Part model, mm, in its own coordinate system. Face numbers are marked on the shaded views. A direction names the side the tool comes from. Give positions to 0.01 mm unless a question says otherwise; leave off trailing zeros. Order: outer loops, then holes, each group sorted by start corner. A loop starts at its lowest first (then second) coordinate and runs counter-clockwise, first axis right, second up. Notation, with made-up numbers: (-38.75, 24.5) - (10.25, 24.5) arc R27 cw to (10.25, 48.5) - close; hole circle Ø5 at (16, 12). An arc over 180 degrees is marked (long way). Use one line per item in the form item = value. Start each with the question number.
1. Drill centre lines: line 1 (Y direction, x = -1, z = 15); line 2 (X direction, y = 2.75, z = -0.5); line 3 (X direction, y = 0.75, z = 12). Where is each one in solid material? Low to high.
2. Band-saw the part on C-C, the plane z = 15. List the corners of the cut face in (x, y), plus the area to 3 significant figures.
3. Pull direction Z, two halves, no side cores. Call the marked faces 1, 2 and 3: +Z half, -Z half, draft (parallel to the pull), parting line (faces both ways), or undercut.
4. Pin check, flat tips, straight feed: P1, Ø3, axis at y = 8.5, z = 13, coming from the +X side; P2, Ø5.5, axis at y = 5, z = 15, coming from the -X side; P3, Ø5, axis at x = 8, y = 1, coming from the +Z side; P4, Ø3, axis at x = 19.5, y = 6, coming from the -Z side. Stop position of each tip, or through.
5. Tool access for the marked faces 4, 5 and 6: list every direction of +Z, -Z, +X, -X, +Y, -Y with a clear straight run to the whole face (end or side of a thin tool).
6. Band-saw the part on B-B, the plane x = -2. List the corners of the cut face in (y, z).
7. Band-saw the part on D-D, the plane x = 15. List the corners of the cut face in (y, z), plus the area to 3 significant figures.
8. Band-saw the part on A-A, the plane y = 5. List the corners of the cut face in (x, z), plus the area to 3 significant figures.
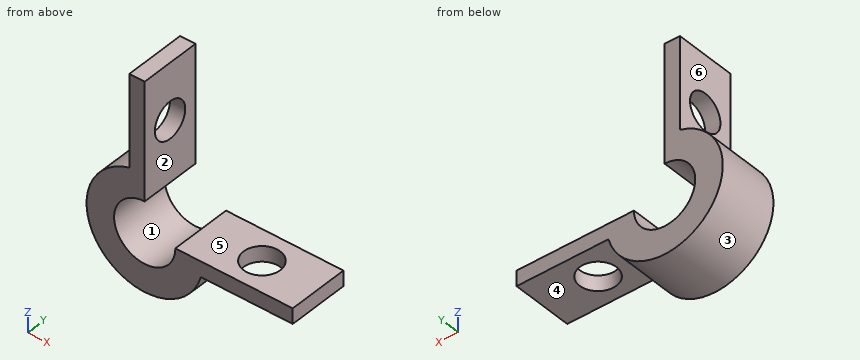
from build123d import *

# Parameters (mm, degrees)
BOSS_EXTRUDE1_DEPTH = 10
SKETCH2_R           = 3
CUT_EXTRUDE1_DEPTH  = 38.349495851
CIRPATTERN1_COUNT   = 2
CIRPATTERN1_ANGLE   = 90


with BuildPart() as part:
    # Sketch1 → Boss-Extrude1 (new body)
    with BuildSketch(Plane(origin=(0, 0, 0), x_dir=(1, 0, 0), z_dir=(0, 1, 0))):
        with BuildLine():
            Line((0, -24.16515139), (0, -5))
            ThreePointArc((0, -5), (-3.535533906, 3.535533906), (5, 0))
            Line((5, 0), (24.16515139, 0))
            Line((24.16515139, 0), (24.16515139, 2.5))
            Line((24.16515139, 2.5), (9.16515139, 2.5))
            ThreePointArc((9.16515139, 2.5), (-6.717514421, 6.717514421), (-2.5, -9.16515139))
            Line((-2.5, -9.16515139), (-2.5, -24.16515139))
            Line((-2.5, -24.16515139), (0, -24.16515139))
        make_face()
    extrude(amount=BOSS_EXTRUDE1_DEPTH)

    # Sketch2 → Cut-Extrude1 (cut, through all)
    with BuildSketch(Plane.ZY.offset(2.5)):
        with Locations((15, 5)):
            Circle(SKETCH2_R)
    cut_extrude1 = extrude(amount=-CUT_EXTRUDE1_DEPTH, mode=Mode.SUBTRACT)

    # CirPattern1: Cut-Extrude1 ×2 about axis
    cirpattern1_axis = Axis((0, 10, 0), (0, 1, 0))
    for i in range(1, CIRPATTERN1_COUNT):
        add(cut_extrude1.rotate(cirpattern1_axis, i * CIRPATTERN1_ANGLE / (CIRPATTERN1_COUNT - 1)), mode=Mode.SUBTRACT)


solid = part.part
From the geometry:
q1.line_1 = 0 to 2, 8 to 10
q1.line_2 = -9.49 to -4.97, 4.97 to 13.02, 16.98 to 24.17
q1.line_3 = -2.5 to 0
q2.outline = (-2.5, 0) - (0, 0) - (0, 2) - (-2.5, 2) - close; (-2.5, 8) - (0, 8) - (0, 10) - (-2.5, 10) - close
q2.area = 10.0 mm²
q3.face_1 = undercut
q3.face_2 = draft
q3.face_3 = parting line
q4.P1 = 0
q4.P2 = through
q4.P3 = 0
q4.P4 = -2.5
q5.face_4 = -Z, +X, +Y, -Y
q5.face_5 = +Z, +X, +Y, -Y
q5.face_6 = +Z, -X, +Y, -Y
q6.outline = (0, -9.29) - (10, -9.29) - (10, -4.58) - (0, -4.58) - close; (0, 4.58) - (10, 4.58) - (10, 24.17) - (0, 24.17) - close; hole circle Ø6 at (5, 15)
q7.outline = (0, -2.5) - (2, -2.5) - (2, 0) - (0, 0) - close; (8, -2.5) - (10, -2.5) - (10, 0) - (8, 0) - close
q7.area = 10.0 mm²
q8.outline = (-2.5, 9.17) arc R9.5 ccw (long way) to (9.17, -2.5) - (12, -2.5) - (12, 0) - (5, 0) arc R5 cw (long way) to (0, 5) - (0, 12) - (-2.5, 12) - close; (-2.5, 18) - (0, 18) - (0, 24.17) - (-2.5, 24.17) - close; (18, -2.5) - (24.17, -2.5) - (24.17, 0) - (18, 0) - close
q8.area = 198 mm²
